Design review of the part built by this model. Coordinates are the model's own, in mm. Coordinates: 2 decimals unless noted, no trailing zeros. Write each loop counter-clockwise with the first axis right and the second up, starting at its lowest first coordinate (ties: lowest second). Pieces come first, ordered by that corner, then holes. Notation, with made-up numbers: (-13.5, 60.5) -> (-3.5, 60.5) arc R12 ccw to (-3.5, 76.5) -> close; hole circle Ø1 at (22.5, -18). An arc over 180 degrees is marked (long way). Answer in a Markdown table with one row per item. Add a question column.
Item 1: To check wall thickness, follow line 1 (Z direction, x = -0.05, y = 0.1); line 2 (X direction, y = 0.05, z = -233); line 3 (Y direction, x = 0.85, z = -60). State the ranges of each line that lie inside material, in increasing order.
Item 2: Take a section at A-A, the plane x = 0. Write out the cut boundary in (y, z).
Item 3: Take a section at B-B, the plane z = -100.5. Write out the cut boundary in (x, y), and give its area (3 significant figures).
from build123d import *

# Parameters (mm, degrees)
SKETCH_1_W      = 2
SKETCH_1_H      = 3
EXTRUDE_1_DEPTH = 0.5
SKETCH_2_W      = 2
SKETCH_2_H      = 3.7
EXTRUDE_2_DEPTH = 0.5
SKETCH_3_R      = 1
EXTRUDE_3_DEPTH = 250
SKETCH_4_R      = 0.5
EXTRUDE_4_DEPTH = 3


with BuildPart() as part:
    # 草图1 → 凸台-拉伸1 (new body)
    with BuildSketch(Plane.XY):
        Rectangle(SKETCH_1_W, SKETCH_1_H)
    extrude(amount=EXTRUDE_1_DEPTH)

    # 草图2 → 凸台-拉伸2 (add)
    with BuildSketch(Plane(origin=(0, 1.5, 0), x_dir=(1, 0, 0), z_dir=(0, 1, 0))):
        with Locations((0, -1.85)):
            Rectangle(SKETCH_2_W, SKETCH_2_H)
    extrude(amount=EXTRUDE_2_DEPTH)

    # 草图3 → 凸台-拉伸3 (add)
    with BuildSketch(Plane(origin=(0, 0, 0), x_dir=(-1, 0, 0), z_dir=(0, 0, -1))):
        Circle(SKETCH_3_R)
    extrude(amount=EXTRUDE_3_DEPTH)

    # 草图4 → 凸台-拉伸4 (add)
    with BuildSketch(Plane.XZ.offset(-1.5)):
        with Locations(Location((0, 2.2, 0), (0, 0, 90))):
            Circle(SKETCH_4_R)
    extrude(amount=EXTRUDE_4_DEPTH)


solid = part.part
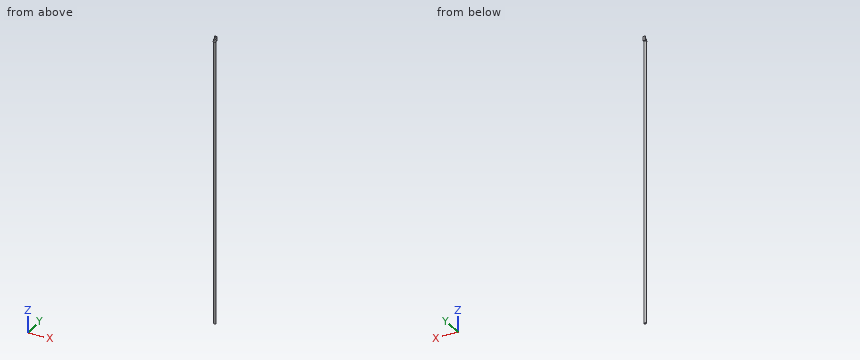
Answers:
| question | item | result |
|---|---|---|
| 1 | line 1 | z = -250 to 0.5, 1.7 to 2.7 |
| 1 | line 2 | x = -1 to 1 |
| 1 | line 3 | y = -0.53 to 0.53 |
| 2 | outline | (-1.5, 0) -> (-1, 0) -> (-1, -250) -> (1, -250) -> (1, 0) -> (2, 0) -> (2, 3.7) -> (1.5, 3.7) -> (1.5, 2.7) -> (-1.5, 2.7) -> (-1.5, 1.7) -> (1.5, 1.7) -> (1.5, 0.5) -> (-1.5, 0.5) -> close |
| 3 | outline | circle Ø2 at (0, 0) |
| 3 | area | 3.14 mm^2 |
